from build123d import *

# Parameters (mm, degrees)
BOSS_EXTRUDE1_DEPTH = 25
BOSS_EXTRUDE2_DEPTH = 1
BOSS_EXTRUDE3_DEPTH = 3


with BuildPart() as part:
    # Sketch2 → Boss-Extrude1 (new body)
    with BuildSketch(Plane.XY):
        Polygon((2.132692592, -1.304462459), (2.196043924, 1.194734734), (0.063351332, 2.499197193), (-2.132692592, 1.304462459), (-2.196043924, -1.194734734), (-0.063351332, -2.499197193), align=None)
    extrude(amount=BOSS_EXTRUDE1_DEPTH)

    # Sketch3 → Boss-Extrude2 (add)
    with BuildSketch(Plane.XY):
        Polygon((2.806699615, -1.572449101), (2.765130676, 1.644448617), (-0.04156894, 3.216897718), (-2.806699615, 1.572449101), (-2.765130676, -1.644448617), (0.04156894, -3.216897718), align=None)
    extrude(amount=-BOSS_EXTRUDE2_DEPTH)

    # Sketch4 → Boss-Extrude3 (add)
    with BuildSketch(Plane.XY):
        Polygon((-2.150386975, -1.275082687), (0.029060512, -2.499831092), (2.179447487, -1.224748404), (2.150386975, 1.275082687), (-0.029060512, 2.499831092), (-2.179447487, 1.224748404), align=None)
    extrude(amount=-BOSS_EXTRUDE3_DEPTH)


solid = part.part
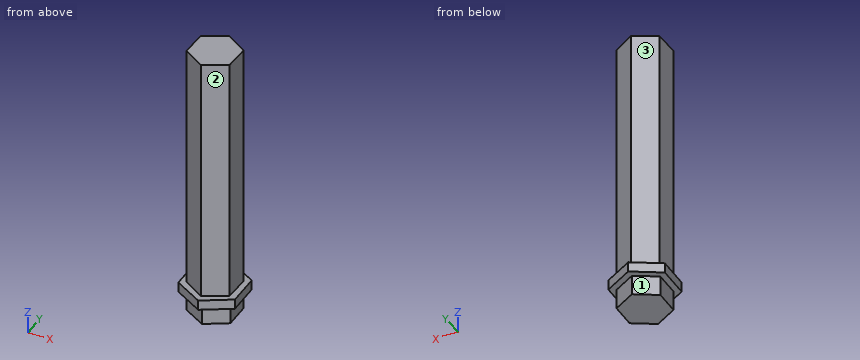
Read the model definition and answer for the solid it produces. Units are mm, in the model's axes. Face numbers are marked on the shaded views. A direction names the side the tool comes from. Round coordinates to 2 decimals unless told otherwise and drop trailing zeros. Write each loop counter-clockwise with the first axis right and the second up, starting at its lowest first coordinate (ties: lowest second). Pieces come first, ordered by that corner, then holes. Notation, with made-up numbers: M -13,36 L 45,36 A19 ccw 45,50 Z; hole C 54,80 d6. An arc over 180 degrees is marked long. Use a Markdown table: item, result.
1) A tool of negligible diameter and unlimited length cuts with its end or side. For the marked faces 1, 2 and 3, from which of +Z, -Z, +X, -X, +Y, -Y can it reach the whole face along a straight path? Write none if from no direction.
Answers follow:
| item | result |
|---|---|
| face 1 | -Z, -X, +Y |
| face 2 | +Z, +X, -Y |
| face 3 | +Z, -X, +Y |
2) The part is cut by section C-C (y = 0.25). Write down the section's boundary in (x, z), plus the area to 3 significant figures.
Answers follow:
| item | result |
|---|---|
| outline | M -2.79,-1 L -2.17,-1 L -2.17,-3 L 2.16,-3 L 2.16,-1 L 2.78,-1 L 2.78,0 L 2.17,0 L 2.17,25 L -2.16,25 L -2.16,0 L -2.79,0 Z |
| area | 123 mm2 |
3) The part is cut by section A-A (x = -1.65). Write down the section's boundary in (y, z), plus the area to 3 significant figures.
Answers follow:
| item | result |
|---|---|
| outline | M -2.27,-1 L -1.56,-1 L -1.56,-3 L 1.54,-3 L 1.54,-1 L 2.26,-1 L 2.26,0 L 1.57,0 L 1.57,25 L -1.53,25 L -1.53,0 L -2.27,0 Z |
| area | 88.1 mm2 |
4) The part is cut by section B-B (z = 9.25). Write down the section's boundary in (x, y).
Answers follow:
| item | result |
|---|---|
| outline | M -2.2,-1.19 L -0.06,-2.5 L 2.13,-1.3 L 2.2,1.19 L 0.06,2.5 L -2.13,1.3 Z |
5) Straight lines are drawn through the part: line 1 along Z through (x, y) = (2.4, -0.75); line 2 along X through (y, z) = (0.75, 6); line 3 along X through (y, z) = (-0.5, 7.5). For each, find the intervals that lie inside material, in ascending order. Write a range as [from, to].
Answers follow:
| item | result |
|---|---|
| line 1 | z = [-1, 0] |
| line 2 | x = [-2.15, 2.18] |
| line 3 | x = [-2.18, 2.15] |
6) Flat-ended cylindrical pins translate along their axes: pin 1 (2 mm diameter, centred on x = -2, z = 3.5, fed in from -Y); pin 2 (3 mm diameter, centred on y = 1, z = 6.5, fed in from +X); pin 3 (3 mm diameter, centred on x = -1, z = 3, fed in from +Y). Find the tip coordinate at first contact, or state that the pin passes through.
Answers follow:
| item | result |
|---|---|
| pin 1 | stops at y = -1.93 |
| pin 2 | stops at x = 2.2 |
| pin 3 | stops at y = 2.5 |
